```python
from build123d import *

# Parameters (mm, degrees)
F1_DEPTH = 25.4


with BuildPart() as f1:
    # F0 (on Front) → F1 (new body)
    with BuildSketch(Plane.XZ):
        with BuildLine():
            add(Edge.make_bspline(
                [(-165.1, -12.7), (-160.657838, 0), (-103.340782, 4.108928), (-69.85, 10.16)],
                knots=[0, 0, 0, 0, 97.954796, 97.954796, 97.954796, 97.954796], degree=3))
            add(Edge.make_bspline(
                [(-165.1, -12.7), (-147.857636, -23.46072), (-135.454967, -21.166667), (-120.63245, -25.4)],
                knots=[0, 0, 0, 0, 46.245572, 46.245572, 46.245572, 46.245572], degree=3))
            Line((-120.63245, -25.4), (-120.63245, -39.115937))
            add(Edge.make_bspline(
                [(-120.63245, -39.115937), (-109.949814, -43.202554), (-101.051494, -40.286522), (-90.506003, -44.45)],
                knots=[0, 0, 0, 0, 30.595017, 30.595017, 30.595017, 30.595017], degree=3))
            Line((-90.506003, -44.45), (-90.49646, -34.296204))
            Line((-90.49646, -34.296204), (-65.09646, -29.478624))
            add(Edge.make_bspline(
                [(151.454941, -20.844295), (76.237051, -25.794228), (10.784542, -28.536206), (-65.09646, -29.478624)],
                knots=[0, 0, 0, 0, 216.723466, 216.723466, 216.723466, 216.723466], degree=3))
            Line((151.454941, -20.844295), (165.1, -11.43))
            Line((165.1, -11.43), (159.076229, 36.646433))
            add(Edge.make_bspline(
                [(152.4, 44.45), (156.209528, 42.954981), (158.982977, 42.765886), (159.076229, 36.646433)],
                knots=[0, 0, 0, 0, 10.269746, 10.269746, 10.269746, 10.269746], degree=3))
            Line((152.4, 44.45), (125.73, 44.45))
            add(Edge.make_bspline(
                [(106.68, 12.7), (110.074804, 15.075844), (120.621224, 34.334068), (125.73, 44.45)],
                knots=[0, 0, 0, 0, 37.026545, 37.026545, 37.026545, 37.026545], degree=3))
            add(Edge.make_bspline(
                [(81.28, 5.08), (82.77345, 5.442668), (98.651765, 7.514939), (106.68, 12.7)],
                knots=[0, 0, 0, 0, 26.518379, 26.518379, 26.518379, 26.518379], degree=3))
            add(Edge.make_bspline(
                [(12.7, 6.35), (54.409864, 3.585023), (80.389956, 3.057459), (81.28, 5.08)],
                knots=[0, 0, 0, 0, 68.591758, 68.591758, 68.591758, 68.591758], degree=3))
            add(Edge.make_bspline(
                [(5.08, 19.05), (9.753358, 15.723685), (10.16, 10.583333), (12.7, 6.35)],
                knots=[0, 0, 0, 0, 14.810618, 14.810618, 14.810618, 14.810618], degree=3))
            add(Edge.make_bspline(
                [(-63.5, 19.05), (-47.14213, 22.504569), (-0.091556, 19.008015), (5.08, 19.05)],
                knots=[0, 0, 0, 0, 68.58, 68.58, 68.58, 68.58], degree=3))
            Line((-63.5, 19.05), (-69.85, 10.16))
        make_face()
    extrude(amount=F1_DEPTH)


solid = f1.part
```
For this review, take the finished solid that the model builds, in its own axes (mm). Give positions to 0.01 mm unless a question says otherwise; leave off trailing zeros.
1) Wall thickness on line 1 (X direction, y = -13.5, z = 14.5); line 2 (Z direction, x = -58, y = -15); line 3 (Z direction, x = -25.5, y = -12.25): over which ranges is each line inside the solid? List them lowest first.
2) Insertion check: pin 1 (12 mm diameter, centred on y = -8.5, z = 16.5, fed in from +X); pin 2 (10 mm diameter, centred on y = -11, z = -3, fed in from +X); pin 3 (3 mm diameter, centred on y = -12, z = 16, fed in from -X). Each pin has a flat end and moves straight along its axis. Give the tip position at first contact, or say it passes through.
3) The part is to be moulded in two halves that separate along X. For faces 1 (the face through (162.13, -12.52, 12.27)), 2 (the face through (2, 0, -9)), 3 (the face through (-120.632, -13, -32)), say which applies: released by +X, released by -X, zero draft, split by the parting line, or undercut.
Derived:
1. line 1: x = -66.75 to 8.98, 108.4 to 161.85
1. line 2: z = -29.38 to 19.86
1. line 3: z = -28.8 to 20.34
2. pin 1: stops at x = 162.35
2. pin 2: stops at x = 164.67
2. pin 3: stops at x = -66.75
3. face 1: released by +X
3. face 2: zero draft
3. face 3: released by -X
